```python
from build123d import *

# Parameters (mm, degrees)
F0_R     = 1.7526
F0_R_2   = 4
F0_W     = 12.7
F0_H     = 5.842
F1_DEPTH = 5.842
F2_R     = 3.175


# Not quite as in the source:
# - a feature names something its author has since deleted; it is built from what else it names


with BuildPart() as f1:
    # F0 (on Front) → F1 (new body)
    with BuildSketch(Plane.XZ):
        Polygon((-12.7, 12.7), (-25.4, 12.7), (-25.4, -12.7), (-19.05, -12.7), (-19.05, -18.542), (-6.35, -18.542), (-6.35, -12.7), (-1.7526, -12.7), (-1.7526, -9.525), (-3.96875, -9.525), (-3.96875, -6.746875), (-1.7526, -6.746875), (-1.7526, -3.571875), (1.7526, -3.571875), (1.7526, -6.746875), (3.96875, -6.746875), (3.96875, -9.525), (1.7526, -9.525), (1.7526, -12.7), (6.35, -12.7), (6.35, -18.542), (19.05, -18.542), (19.05, -12.7), (25.4, -12.7), (25.4, 12.7), (12.7, 12.7), align=None)
        with Locations((-19.05, -8.255)):
            Circle(F0_R, mode=Mode.SUBTRACT)
        with Locations((19.05, -8.255)):
            Circle(F0_R, mode=Mode.SUBTRACT)
        with Locations((-19.05, 0)):
            Circle(F0_R_2, mode=Mode.SUBTRACT)
        with Locations((-1, 3.175)):
            Rectangle(F0_W, F0_H, mode=Mode.SUBTRACT)
        with Locations((-19.05, 8.255)):
            Circle(F0_R, mode=Mode.SUBTRACT)
        with Locations((19.05, 0)):
            Circle(F0_R_2, mode=Mode.SUBTRACT)
        with Locations((19.05, 8.255)):
            Circle(F0_R, mode=Mode.SUBTRACT)
    extrude(amount=F1_DEPTH)

    # F2
    f2_edges = [f1.edges().sort_by_distance(p)[0] for p in [
        (-25.4, -2.921, 12.7),
        (25.4, -2.921, 12.7),
    ]]
    fillet(f2_edges, radius=F2_R)


solid = f1.part
```
Design review of the part built by this model. Coordinates are the model's own, in mm. A direction names the side the tool comes from. Coordinates: 2 decimals unless noted, no trailing zeros. Order: outer loops, then holes, each group sorted by start corner. A loop starts at its lowest first (then second) coordinate and runs counter-clockwise, first axis right, second up. Notation, with made-up numbers: (57.25, 67.5) -> (84.25, 67.5) arc R37 ccw to (84.25, 103.5) -> close; hole circle Ø7 at (-20, 46). An arc over 180 degrees is marked (long way). One line per item, written item: value. Start each with the question number.
Q1. Take a section at A-A, the plane x = 0.5. State the section outline as (y, z) points.
Q2. Tool access review of faces 5 (the flat face through (1.753, -3, -5)), 6 (the flat face through (19.05, -3, -16)), 7 (the flat face through (-3.969, -3, -8)): name each direction out of +Z, -Z, +X, -X, +Y, -Y from which nothing blocks a thin tool from reaching the whole face with its end or side.
Q3. Mouldability with a two-part tool opening along Z and no side actions: class faces 1 (the cylindrical face through (17.3, -2.9, -8.2)), 2 (the flat face through (-1.753, -3, -5)), 3 (the cylindrical face through (-23.046, -2.88, 0.176)), 4 (the flat face through (4, -3, -12.7)) as pulls with the +Z half, pulls with the -Z half, needs draft (parallel to the pull), parting line crosses it, or undercut.
Q4. Take a section at B-B, the plane y = -4.2. Give the number of separate pieces and of enclosed holes in the cut face, then the cut area to 3 significant figures.
Q5. Insertion check: pin 1 Ø1.1 at (x, y) = (-2.5, -3) entering from -Z; pin 2 Ø3 at (y, z) = (-3.5, -15.5) entering from -X. Each pin has a flat end and moves straight along its axis. Give the tip position at first contact, or say it passes through.
Q6. For probe 1 along Z at (x, y) = (-3.5, -3.4) (3 decimals); probe 2 along Z at (x, y) = (-4, -2.3); probe 3 along X at (y, z) = (-4.7, -13), list the stretches that pass through material, from the lowest coordinate up.
Values follow:
1. outline: (-5.84, -3.57) -> (0, -3.57) -> (0, 0.25) -> (-5.84, 0.25) -> close; (-5.84, 6.1) -> (0, 6.1) -> (0, 12.7) -> (-5.84, 12.7) -> close
2. face 5: -Z, +Y, -Y
2. face 6: -Z, +X, +Y, -Y
2. face 7: +Y, -Y
3. face 1: undercut
3. face 2: needs draft
3. face 3: undercut
3. face 4: pulls with the -Z half
4. separate pieces: 1
4. enclosed holes: 7
4. area: 1,180 mm2
5. pin 1: stops at z = -12.7
5. pin 2: stops at x = -19.05
6. probe 1: z = -12.7 to -9.525, -6.747 to 0.254, 6.096 to 12.7
6. probe 2: z = -12.7 to 0.25, 6.1 to 12.7
6. probe 3: x = -19.05 to -6.35, 6.35 to 19.05
